from build123d import *

# Parameters (mm, degrees)
SKETCH1_R           = 17
BOSS_EXTRUDE1_DEPTH = 25
SKETCH1_3_R         = 19
BOSS_EXTRUDE2_DEPTH = 8
BOSS_EXTRUDE3_DEPTH = 15
SKETCH3_R           = 16
BOSS_EXTRUDE4_DEPTH = 15
SKETCH4_R           = 16
BOSS_EXTRUDE5_DEPTH = 5
BOSS_EXTRUDE6_DEPTH = 15
SKETCH6_R           = 16
BOSS_EXTRUDE7_DEPTH = 15
BOSS_EXTRUDE8_START = 2.5
SKETCH7_R           = 17
BOSS_EXTRUDE8_DEPTH = 2.5


with BuildPart() as part:
    # Sketch1 → Boss-Extrude1 (new body)
    with BuildSketch(Plane.XY):
        Circle(SKETCH1_R)
    extrude(amount=-BOSS_EXTRUDE1_DEPTH)

    # Sketch1<3> → Boss-Extrude2 (add)
    with BuildSketch(Plane.XY):
        Circle(SKETCH1_3_R)
    extrude(amount=BOSS_EXTRUDE2_DEPTH)

    # Sketch2 → Boss-Extrude3 (add)
    with BuildSketch(Plane.XY.offset(8)):
        with BuildLine():
            ThreePointArc((-9.986058572, 41.752758122), (3.989062652, 45.958951954), (17.330326456, 40.042300883))
            ThreePointArc((17.330326456, 40.042300883), (35.227782907, 15.421350298), (43.89459329, -13.757350031))
            ThreePointArc((43.89459329, -13.757350031), (-0.356861624, -45.998615738), (-44.102758556, -13.074658228))
            ThreePointArc((-44.102758556, -13.074658228), (-32.131083622, 17.504265061), (-9.986058572, 41.752758122))
        make_face()
    boss_extrude3 = extrude(amount=BOSS_EXTRUDE3_DEPTH)

    # Sketch3 → Boss-Extrude4 (add)
    with BuildSketch(Plane.XY.offset(23)):
        with Locations((3.010021098, 25.549805608)):
            Circle(SKETCH3_R)
    boss_extrude4 = extrude(amount=BOSS_EXTRUDE4_DEPTH)

    # Mirror1: Boss-Extrude3, Boss-Extrude4 across plane
    add(boss_extrude3.mirror(Plane(origin=(3.010021098, 25.549805608, 38), x_dir=(1, 0, 0), z_dir=(0, 0, 1))))
    add(boss_extrude4.mirror(Plane(origin=(3.010021098, 25.549805608, 38), x_dir=(1, 0, 0), z_dir=(0, 0, 1))))

    # Sketch4 → Boss-Extrude5 (add)
    with BuildSketch(Plane.XY.offset(68)):
        Circle(SKETCH4_R)
    extrude(amount=BOSS_EXTRUDE5_DEPTH)

    # Sketch5 → Boss-Extrude6 (add)
    with BuildSketch(Plane.XY.offset(73)):
        with BuildLine():
            ThreePointArc((-17.330326456, -40.042300883), (-3.989062652, -45.958951954), (9.986058572, -41.752758122))
            ThreePointArc((9.986058572, -41.752758122), (32.131083622, -17.504265061), (44.102758556, 13.074658228))
            ThreePointArc((44.102758556, 13.074658228), (0.356861624, 45.998615738), (-43.89459329, 13.757350031))
            ThreePointArc((-43.89459329, 13.757350031), (-35.227782907, -15.421350298), (-17.330326456, -40.042300883))
        make_face()
    boss_extrude6 = extrude(amount=BOSS_EXTRUDE6_DEPTH)

    # Sketch6 → Boss-Extrude7 (add)
    with BuildSketch(Plane.XY.offset(88)):
        with Locations((-2.406352883, -26.965307304)):
            Circle(SKETCH6_R)
    boss_extrude7 = extrude(amount=BOSS_EXTRUDE7_DEPTH)

    # Mirror2: Boss-Extrude6, Boss-Extrude7 across plane
    add(boss_extrude6.mirror(Plane(origin=(-2.406352883, -26.965307304, 103), x_dir=(1, 0, 0), z_dir=(0, 0, 1))))
    add(boss_extrude7.mirror(Plane(origin=(-2.406352883, -26.965307304, 103), x_dir=(1, 0, 0), z_dir=(0, 0, 1))))

    # Sketch7 → Boss-Extrude8 (add)
    with BuildSketch(Plane.XY.offset(133).offset(BOSS_EXTRUDE8_START)):
        Circle(SKETCH7_R)
    extrude(amount=-BOSS_EXTRUDE8_DEPTH)

    # Mirror3: part across plane


with BuildPart() as part_1:
    add(part.part)
    add(part.part.mirror(Plane.XY.offset(135.5)))


solid = part_1.part
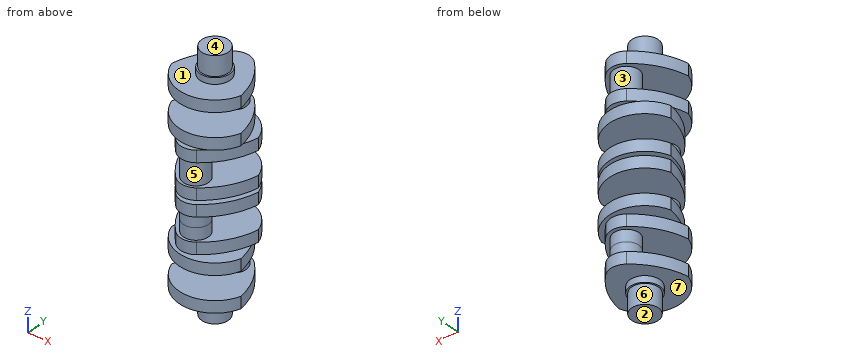
Model file for the job. Use its own axes, mm. Face numbers are marked on the shaded views. A direction names the side the tool comes from. Coordinates: 2 decimals unless noted, no trailing zeros. Write each loop counter-clockwise with the first axis right and the second up, starting at its lowest first coordinate (ties: lowest second). Pieces come first, ordered by that corner, then holes. Notation, with made-up numbers: (35, 20.5) - (64, 20.5) arc R28 cw to (64, 51.5) - close; hole circle Ø9 at (12, 61). An arc over 180 degrees is marked (long way). Write each question's results on one line, items separated by ' | '. Start each with the question number.
1) Probe line 1 along Z through (x, y) = (18.5, 29); line 2 along Z through (x, y) = (36.5, -22); line 3 along Z through (x, y) = (-39, 9.5). List the from-to ranges inside material, lowest first. Write a range as from..to.
2) Flat gauge pins, fed straight in: P1, Ø4, axis at x = -30.5, z = 196, coming from the +Y side; P2, Ø3, axis at x = -2.5, z = 182, coming from the +Y side; P3, Ø1, axis at x = -21, y = -18, coming from the -Z side. Where does each tip first touch, or does it go through?
3) Cut at D-D (z = 168.5). Write the cut outline in (x, y), then the cut area to 3 significant figures.
4) Mould opens along Z. For the marked faces 4, 5, 6 and 7 say: pulls with the +Z half, pulls with the -Z half, needs draft (parallel to the pull), parting line crosses it, or undercut.
5) Cut at A-A (x = -39). Count the separate pieces of the cut face and the enclosed holes in it, then the cut area to 3 significant figures.
6) 3-axis set-ups, long thin cutter, end or side, ignore diameter. For the marked faces 1, 2 and 3: which of +Z, -Z, +X, -X, +Y, -Y reach the whole face in a straight line?
Returned:
1) line 1: 8..68, 73..88, 118..133, 138..153, 183..198, 203..263 | line 2: 8..23, 53..68, 203..218, 248..263 | line 3: 73..88, 118..133, 138..153, 183..198
2) P1: y = 36.11 | P2: y = 45.98 | P3: z = 8
3) outline: circle Ø32 at (-2.41, -26.97) | area: 804 mm^2
4) face 4: pulls with the +Z half | face 5: undercut | face 6: needs draft | face 7: pulls with the -Z half
5) separate pieces: 8 | enclosed holes: 0 | area: 3,570 mm^2
6) face 1: +Z | face 2: -Z, +X, -X, +Y, -Y | face 3: none
